from build123d import *

# Parameters (mm, degrees)
SKETCH1_R               = 5
BOSS_EXTRUDE1_DEPTH     = 15
CUT_EXTRUDE1_REACH      = 18.583
CUT_EXTRUDE1_END_RADIUS = 5
SKETCH3_R               = 1.5
SKETCH4_R               = 5
BOSS_EXTRUDE2_DEPTH     = 2
BOSS_EXTRUDE3_DEPTH     = 25


with BuildPart() as part:
    # Sketch1 → Boss-Extrude1 (new body)
    with BuildSketch(Plane.XY):
        Circle(SKETCH1_R)
        with BuildLine():
            Line((-1.656238208, 2.65), (1.656238208, 2.65))
            ThreePointArc((1.656238208, 2.65), (0, -3.125), (-1.656238208, 2.65))
        make_face(mode=Mode.SUBTRACT)
    extrude(amount=BOSS_EXTRUDE1_DEPTH)

    # Cut-Extrude1: up to this cylinder (the profile starts inside it)
    cut_extrude1_end = Plane(origin=(0, 0, 5), z_dir=(0, 0, -1)) * Cylinder(CUT_EXTRUDE1_END_RADIUS, 48.166, mode=Mode.PRIVATE)
    # Sketch3 → Cut-Extrude1 (cut, up to the surface)
    with BuildSketch(Plane(origin=(0, 0, 0), x_dir=(1, 0, 0), z_dir=(0, 1, 0)), mode=Mode.PRIVATE) as cut_extrude1_sk1:
        with Locations(Location((0, -5, 0), (0, 0, 90))):
            Circle(SKETCH3_R)
    cut_extrude1_tool1 = extrude(cut_extrude1_sk1.sketch, amount=CUT_EXTRUDE1_REACH, mode=Mode.PRIVATE) & cut_extrude1_end
    add(cut_extrude1_tool1.solids().sort_by_distance((0, 0, 5))[0], mode=Mode.SUBTRACT)

    # Sketch4 → Boss-Extrude2 (add)
    with BuildSketch(Plane.XY.offset(15)):
        Circle(SKETCH4_R)
    extrude(amount=BOSS_EXTRUDE2_DEPTH)

    # Sketch6 → Boss-Extrude3 (add)
    with BuildSketch(Plane.XY.offset(17)):
        with BuildLine():
            Line((1.71537168, 2.4), (-1.71537168, 2.4))
            ThreePointArc((-1.71537168, 2.4), (-1.349472776, -2.623246696), (2.95, 0))
            ThreePointArc((2.95, 0), (2.623246696, 1.349472776), (1.71537168, 2.4))
        make_face()
    extrude(amount=BOSS_EXTRUDE3_DEPTH)


solid = part.part
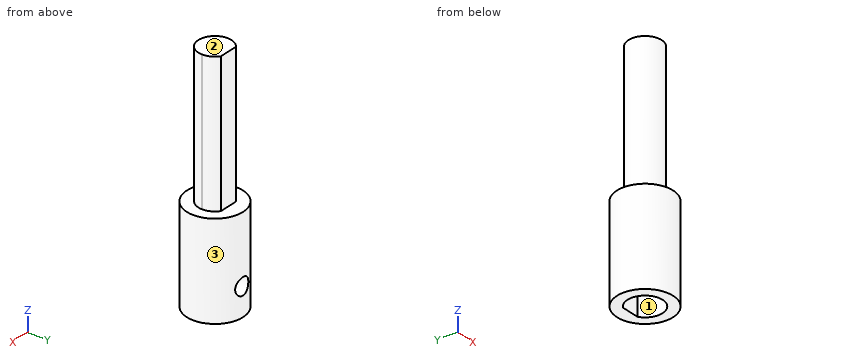
Can you work these out from the model? Positions are in its coordinate system, mm. Face numbers are marked on the shaded views. Coordinates: 2 decimals unless noted, no trailing zeros. Write each loop counter-clockwise with the first axis right and the second up, starting at its lowest first coordinate (ties: lowest second). Pieces come first, ordered by that corner, then holes. Notation, with made-up numbers: (16, 7) -> (65, 7) arc R21 ccw to (65, 16) -> close; hole circle Ø3 at (89, -4.5). An arc over 180 degrees is marked (long way). Write each question's results on one line, items separated by ' | '. Start each with the question number.
Q1. Imagine slicing it at B-B (y = 1.5). Write out the boundary of the cut face in (x, z).
Q2. Imagine slicing it at A-A (x = 0). Write out the boundary of the cut face in (y, z) (3 decimals).
Q3. We'd pull the mould along X, two halves only. Please class the marked faces 1, 2 and 3: +X half, -X half, draft (parallel to the pull), parting line (faces both ways), or undercut.
Q4. Imagine slicing it at D-D (y = 3.5). Write out the boundary of the cut face in (x, z).
Q5. Imagine slicing it at C-C (z = 21). Write out the boundary of the cut face in (x, y), then the cut area to 3 significant figures.
Q6. I'm going to push flat-ended pins straight in: pin 1 (3 mm diameter, centred on x = -1, z = 31, fed in from +Y); pin 2 (5 mm diameter, centred on x = 0, y = 0, fed in from -Z); pin 3 (5 mm diameter, centred on y = 1, z = 25.5, fed in from +X). Where does each tip first touch, or does it pass through?
Q7. If I drill on probe 1 along Y at (x, z) = (0, 14) (3 decimals); probe 2 along Z at (x, y) = (3.25, 1.75); probe 3 along Z at (x, y) = (-1.25, 1), over which ranges is the centre line in solid material (lowest first)?
Taken from the geometry:
1) outline: (-4.77, 0) -> (-2.74, 0) -> (-2.74, 15) -> (2.74, 15) -> (2.74, 0) -> (4.77, 0) -> (4.77, 17) -> (2.54, 17) -> (2.54, 42) -> (-2.54, 42) -> (-2.54, 17) -> (-4.77, 17) -> close
2) outline: (-5, 0) -> (-3.125, 0) -> (-3.125, 15) -> (2.65, 15) -> (2.65, 6.5) -> (5, 6.5) -> (5, 17) -> (2.4, 17) -> (2.4, 42) -> (-2.95, 42) -> (-2.95, 17) -> (-5, 17) -> close; (2.65, 0) -> (5, 0) -> (5, 3.5) -> (2.65, 3.5) -> close
3) face 1: undercut | face 2: draft | face 3: parting line
4) outline: (-3.57, 0) -> (3.57, 0) -> (3.57, 17) -> (-3.57, 17) -> close; hole circle Ø3 at (0, 5)
5) outline: (-1.72, 2.4) arc R2.95 ccw (long way) to (1.72, 2.4) -> close | area: 26.1 mm^2
6) pin 1: stops at y = 2.4 | pin 2: stops at z = 15 | pin 3: stops at x = 2.95
7) probe 1: y = -5 to -3.125, 2.65 to 5 | probe 2: z = 0 to 17 | probe 3: z = 15 to 42
